from build123d import *

# Parameters (mm, degrees)
F0_R     = 10
F1_DEPTH = 10
F3_DEPTH = 10
F5_DEPTH = 10
F6_R     = 17
F6_R_2   = 10
F7_DEPTH = 2.5


with BuildPart() as f1:
    # F0 (on Top) → F1 (new body)
    with BuildSketch(Plane.XY):
        with BuildLine():
            Line((13.2287565553, 0), (0, 0))
            Line((0, 0), (-13.2287565553, 0))
            ThreePointArc((-13.2287565553, 0), (-20, -15), (-13.2287565553, -30))
            Line((-13.2287565553, -30), (13.2287565553, -30))
            ThreePointArc((13.2287565553, -30), (18.2287565553, -23.2287565553), (20, -15))
            ThreePointArc((20, -15), (18.2287565553, -6.7712434447), (13.2287565553, 0))
        make_face()
        with Locations((0, -15)):
            Circle(F0_R, mode=Mode.SUBTRACT)
        with BuildLine():
            Line((-13.2287565553, 0), (0, 0))
            Line((0, 0), (13.2287565553, 0))
            ThreePointArc((13.2287565553, 0), (0, 5), (-13.2287565553, 0))
        make_face()
        with BuildLine():
            ThreePointArc((-13.2287565553, -30), (-20, -15), (-13.2287565553, 0))
            Line((-13.2287565553, 0), (-30, 0))
            Line((-30, 0), (-30, -30))
            Line((-30, -30), (-13.2287565553, -30))
        make_face()
        with BuildLine():
            Line((30, 0), (13.2287565553, 0))
            ThreePointArc((13.2287565553, 0), (18.2287565553, -6.7712434447), (20, -15))
            ThreePointArc((20, -15), (18.2287565553, -23.2287565553), (13.2287565553, -30))
            Line((13.2287565553, -30), (30, -30))
            Line((30, -30), (30, 0))
        make_face()
        with BuildLine():
            Line((13.2287565553, -30), (-13.2287565553, -30))
            ThreePointArc((-13.2287565553, -30), (0, -35), (13.2287565553, -30))
        make_face()
    extrude(amount=F1_DEPTH)

    # F2 (on face) → F3 (join)
    with BuildSketch(Plane.YZ.offset(30)):
        with BuildLine():
            Line((-30, 30), (-30, 10))
            Line((-30, 10), (0, 10))
            Line((0, 10), (0, 30))
            Line((0, 30), (-7.5, 30))
            ThreePointArc((-7.5, 30), (-15, 22.5), (-22.5, 30))
            Line((-22.5, 30), (-30, 30))
        make_face()
        with BuildLine():
            ThreePointArc((0, 30), (-15, 45), (-30, 30))
            Line((-30, 30), (-22.5, 30))
            ThreePointArc((-22.5, 30), (-15, 37.5), (-7.5, 30))
            Line((-7.5, 30), (0, 30))
        make_face()
    extrude(amount=-F3_DEPTH)

    # F4 (on face) → F5 (join)
    with BuildSketch(Plane(origin=(-30, 0, 0), x_dir=(0, -1, 0), z_dir=(-1, 0, 0))):
        with BuildLine():
            Line((0, 30), (0, 10))
            Line((0, 10), (30, 10))
            Line((30, 10), (30, 30))
            Line((30, 30), (22.5, 30))
            ThreePointArc((22.5, 30), (15, 22.5), (7.5, 30))
            Line((7.5, 30), (0, 30))
        make_face()
        with BuildLine():
            ThreePointArc((30, 30), (15, 45), (0, 30))
            Line((0, 30), (7.5, 30))
            ThreePointArc((7.5, 30), (15, 37.5), (22.5, 30))
            Line((22.5, 30), (30, 30))
        make_face()
    extrude(amount=-F5_DEPTH)

    # F6 (on face) → F7 (join)
    with BuildSketch(Plane(origin=(0, 0, 0), x_dir=(1, 0, 0), z_dir=(0, 0, -1))):
        with Locations((0, 15)):
            Circle(F6_R)
        with Locations((0, 15)):
            Circle(F6_R_2, mode=Mode.SUBTRACT)
    extrude(amount=F7_DEPTH)


solid = f1.part
Geometry check sheet. Reference: the model listing, model coordinates, mm. A direction names the side the tool comes from. Give positions to 0.01 mm unless a question says otherwise; leave off trailing zeros. Order: outer loops, then holes, each group sorted by start corner. A loop starts at its lowest first (then second) coordinate and runs counter-clockwise, first axis right, second up.
1. Draft check along X on faces 4 (the face through (0, -35, 5)), 5 (the face through (-20, -15, 20)), 6 (the face through (-1.302, -24.915, 3.838)), 7 (the face through (7.3, -7.7, -2.5)). Enter one of: pulls with the +X half, pulls with the -X half, needs draft (parallel to the pull), parting line crosses it, or undercut.
Completed:
face 4: parting line crosses it
face 5: undercut
face 6: undercut
face 7: needs draft
2. Sectioned sample at A-A (y = -15). Record the boundary of the cut face in (x, z), then the cut area to 3 significant figures.
Completed:
outline: (-30, 0) - (-17, 0) - (-17, -2.5) - (-10, -2.5) - (-10, 10) - (-20, 10) - (-20, 22.5) - (-30, 22.5) - close; (-30, 37.5) - (-20, 37.5) - (-20, 45) - (-30, 45) - close; (10, -2.5) - (17, -2.5) - (17, 0) - (30, 0) - (30, 22.5) - (20, 22.5) - (20, 10) - (10, 10) - close; (20, 37.5) - (30, 37.5) - (30, 45) - (20, 45) - close
area: 835 mm2
3. Depth check by flat-ended pin: pin 1 (13.5 mm diameter, centred on x = 21, z = 12, fed in from -Y); pin 2 (18.5 mm diameter, centred on x = -21.5, z = 10.5, fed in from +Y); pin 3 (5 mm diameter, centred on x = 23.5, z = 9.5, fed in from +Y). Enter the tip coordinate at first touch or a pass-through.
Completed:
pin 1: stops at y = -30
pin 2: stops at y = 0.8
pin 3: stops at y = 0
4. Access from +Z, -Z, +X, -X, +Y, -Y to the whole of each face (thin tool, end or side, straight path). Record for faces 1 (the face through (20, -15, 20)), 2 (the face through (-3.685, 1.596, -1.232)), 3 (the face through (24, -30, 12)).
Completed:
face 1: +Z, +Y, -Y
face 2: -Z
face 3: +Z, -Z, +X, -Y
5. Sectioned sample at B-B (z = 14). Record the boundary of the cut face in (x, y).
Completed:
outline: (-30, -30) - (-20, -30) - (-20, 0) - (-30, 0) - close; (20, -30) - (30, -30) - (30, 0) - (20, 0) - close
6. Scan lines: line 1 (X direction, y = -23.5, z = 31.5); line 2 (Y direction, x = 0, z = 3); line 3 (Z direction, x = -27, y = -15). Record each from-to range of solid material in increasing order.
Completed:
line 1: x = -30 to -20, 20 to 30
line 2: y = -35 to -25, -5 to 5
line 3: z = 0 to 22.5, 37.5 to 45
7. Sectioned sample at D-D (x = -15). Record the boundary of the cut face in (y, z), then the cut area to 3 significant figures.
Completed:
outline: (-30, 0) - (-23, 0) - (-23, -2.5) - (-7, -2.5) - (-7, 0) - (0, 0) - (0, 10) - (-30, 10) - close
area: 340 mm2
8. Sectioned sample at C-C (x = 0). Record the boundary of the cut face in (y, z), then the cut area to 3 significant figures.
Completed:
outline: (-35, 0) - (-32, 0) - (-32, -2.5) - (-25, -2.5) - (-25, 10) - (-35, 10) - close; (-5, -2.5) - (2, -2.5) - (2, 0) - (5, 0) - (5, 10) - (-5, 10) - close
area: 235 mm2
